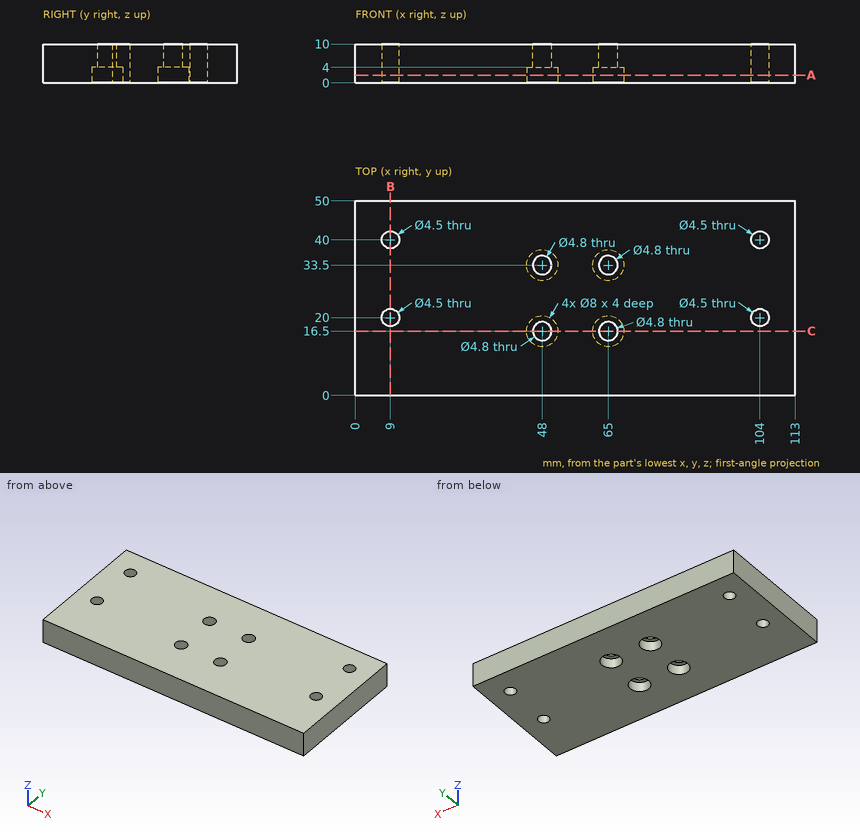
Can you work these out from the drawing? Everything is in mm from the part's minimum corner. Coordinates: 2 decimals unless noted, no trailing zeros. Loops run counter-clockwise (first coordinate to the right, second up) from the corner with the lowest first, then second, coordinate; pieces in that order, holes last.
1) Imagine slicing it at C-C on y = 16.5. List the corners of the cut face in (x, z) for me.
2) I need wall thicknesses on probe 1 along Y at (x, z) = (48, 6.95); probe 2 along Y at (x, z) = (65, 1.05). Which ranges of each line are inside material? Lowest first, please.
3) Imagine slicing it at B-B on x = 9. List the corners of the cut face in (y, z) for me, plus the area to 3 significant figures.
4) Imagine slicing it at A-A on z = 2. State how many separate pieces and enclosed holes the cut face has, plus the area to 3 significant figures.
5) For pin 1 (5 mm diameter, centred on x = 48, y = 33.5, fed in from -Z), with a flat end and sliding along its axis, tell me the tip position at first contact or that it passes through.
Completed:
1. outline: (0, 0) - (44, 0) - (44, 4) - (45.6, 4) - (45.6, 10) - (0, 10) - close; (50.4, 4) - (52, 4) - (52, 0) - (61, 0) - (61, 4) - (62.6, 4) - (62.6, 10) - (50.4, 10) - close; (67.4, 4) - (69, 4) - (69, 0) - (113, 0) - (113, 10) - (67.4, 10) - close
2. probe 1: y = 0 to 14.1, 18.9 to 31.1, 35.9 to 50
2. probe 2: y = 0 to 12.5, 20.5 to 29.5, 37.5 to 50
3. outline: (0, 0) - (17.75, 0) - (17.75, 10) - (0, 10) - close; (22.25, 0) - (37.75, 0) - (37.75, 10) - (22.25, 10) - close; (42.25, 0) - (50, 0) - (50, 10) - (42.25, 10) - close
3. area: 410 mm2
4. separate pieces: 1
4. enclosed holes: 8
4. area: 5,390 mm2
5. pin 1: stops at z = 4
